Source: CAD feature listing. Evaluate the final solid. Frame: model axes, mm. A direction names the side the tool comes from. Round coordinates to 2 decimals unless told otherwise and drop trailing zeros. Order: outer loops, then holes, each group sorted by start corner. A loop starts at its lowest first (then second) coordinate and runs counter-clockwise, first axis right, second up. Notation, with made-up numbers: (27.5, 73.5) - (59.5, 73.5) arc R24 cw to (59.5, 109.5) - close; hole circle Ø5 at (5, 5.25). An arc over 180 degrees is marked (long way). Return JSON: item names as keys, results as strings. Group by question number.
1) Contact query for flat-ended pins moving along their axis: P1, Ø5.5, axis at x = 0, y = -5, coming from the +Z side; P2, Ø5, axis at x = 2, y = -7, coming from the -Z side; P3, Ø2, axis at y = -3, z = -3.5, coming from the +X side. Output: stop coordinate, or through.
2) Section A-A, the plane x = 0.5. Return loops of the section in (y, z) (3 decimals).
3) Section D-D, the plane y = -6. Return loops of the section in (x, z).
4) Ray query, line 1 (Y direction, x = 0.5, z = -2.2) (3 decimals); line 2 (Y direction, x = 0.5, z = 3.25); line 3 (X direction, y = -5, z = 2.75). Return the intervals inside material, ascending. Write a range as from..to.
5) Access query for faces 5 (the flat face through (4, -9, -0.964)), 6 (the flat face through (-3.3, -7.4, -6.214)). Directions: +Z, -Z, +X, -X, +Y, -Y. A direction counts if a zero-diameter tool reaches every point of the face in a straight line with its end or side. Return the directions, or none.
6) Mould query, pull axis Y, two halves, no side actions, for faces 1 (the cylindrical face through (-0.69, -12.87, 2.33)), 2 (the flat face through (0, -15, 0)), 3 (the flat face through (-13.75, -7, 3)), 4 (the flat face through (0, 0, 0)). Classes: pulls with the +Y half, pulls with the -Y half, needs draft (parallel to the pull), parting line crosses it, or undercut.
7) Section B-B, the plane y = -7.5. Return loops of the section in (x, z) (3 decimals).
8) Section C-C, the plane z = -4.5. Return loops of the section in (x, y) (3 decimals).
```python
from build123d import *

# Parameters (mm, degrees)
F1_DEPTH       = 15
F3_D           = 6.95
F3_CBORE_D     = 11
F3_CBORE_DEPTH = 6.5


with BuildPart() as f1:
    # F0 (on Front) → F1 (new body)
    with BuildSketch(Plane.XZ):
        with BuildLine():
            Line((13.75, 5.535829), (-13.75, 5.535829))
            Line((-13.75, 5.535829), (-13.75, -0.214171))
            Line((-13.75, -0.214171), (-7.75, -6.214171))
            Line((-7.75, -6.214171), (8.757582, -6.214171))
            ThreePointArc((8.757582, -6.214171), (10.471279, -0.938491), (13.75, 3.535829))
            Line((13.75, 3.535829), (13.75, 5.535829))
        make_face()
    extrude(amount=F1_DEPTH)

    # F3 (through all)
    with Locations(Plane.XY.offset(5.535829)):
        with Locations((0.5, -7.5)):
            CounterBoreHole(F3_D / 2, F3_CBORE_D / 2, F3_CBORE_DEPTH)


solid = f1.part
```
Geometry check:
{
 "1": {"P1": "z = -0.96", "P2": "z = -6.21", "P3": "x = 9.77"},
 "2": {"outline": "(-15, -6.214) - (-10.975, -6.214) - (-10.975, -0.964) - (-13, -0.964) - (-13, 5.536) - (-15, 5.536) - close; (-4.025, -6.214) - (0, -6.214) - (0, 5.536) - (-2, 5.536) - (-2, -0.964) - (-4.025, -0.964) - close"},
 "3": {"outline": "(-13.75, -0.21) - (-7.75, -6.21) - (-2.63, -6.21) - (-2.63, -0.96) - (-4.79, -0.96) - (-4.79, 5.54) - (-13.75, 5.54) - close; (3.63, -6.21) - (8.76, -6.21) arc R17.5 cw to (13.75, 3.54) - (13.75, 5.54) - (5.79, 5.54) - (5.79, -0.96) - (3.63, -0.96) - close"},
 "4": {"line 1": "-15..-10.975, -4.025..0", "line 2": "-15..-13, -2..0", "line 3": "-13.75..-4.4, 5.4..13"},
 "5": {"face 5": "+Z", "face 6": "-Z, +X, -X, +Y, -Y"},
 "6": {"face 1": "undercut", "face 2": "pulls with the -Y half", "face 3": "needs draft", "face 4": "pulls with the +Y half"},
 "7": {"outline": "(-13.75, -0.214) - (-7.75, -6.214) - (-2.975, -6.214) - (-2.975, -0.964) - (-5, -0.964) - (-5, 5.536) - (-13.75, 5.536) - close; (3.975, -6.214) - (8.758, -6.214) arc R17.5 cw to (13.75, 3.536) - (13.75, 5.536) - (6, 5.536) - (6, -0.964) - (3.975, -0.964) - close"},
 "8": {"outline": "(-9.464, -15) - (9.114, -15) - (9.114, 0) - (-9.464, 0) - close; hole circle Ø6.95 at (0.5, -7.5)"}
}
